Input: part model. Units: mm. Frame: model coordinates. Face numbers are marked on the shaded views. A direction names the side the tool comes from. Coordinates: 2 decimals unless noted, no trailing zeros. Loops run counter-clockwise (first coordinate to the right, second up) from the corner with the lowest first, then second, coordinate; pieces in that order, holes last. Notation, with made-up numbers: (48, -26) -> (94, -26) arc R20 cw to (94, -20) -> close; hole circle Ø3 at (16, -14.75). An arc over 180 degrees is marked (long way). Answer as a JSON object with one key per item and string values.
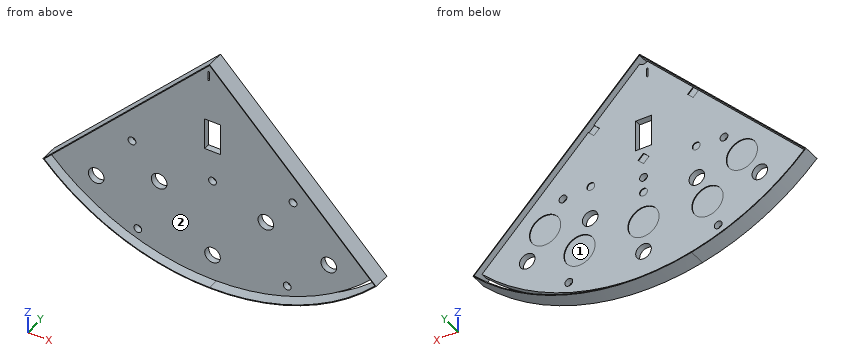
Autodesk Inventor part; units mm, degrees
ref_plane "YZ Plane" through (0, 0, 0) normal (1, 0, 0) x (0, 1, 0)
ref_plane "XZ Plane" through (0, 0, 0) normal (0, 1, 0) x (-1, 0, 0)
ref_plane "XY Plane" through (0, 0, 0) normal (0, 0, 1) x (1, 0, 0)
sketch "草圖1" plane through (0, 0, 0) normal (0, 1, 0) x (-1, 0, 0)
  line L0 (0, 0) -> (-1060.6602, -1060.6602)
  arc A0 (-1060.6602, -1060.6602) -> (0, -1500) centre (0, 0) ccw
  line L1 (0, -1500) -> (0, 0)
  line L2 (0, 0) -> (1060.6602, -1060.6602)
  arc A1 (0, -1500) -> (1060.6602, -1060.6602) centre (0, 0) ccw
  line L3 (1067.7254, -1060.6543) -> (0, 7.0711)
  line L4 (0, 7.0711) -> (-1067.7254, -1060.6543)
  arc A2 (-1067.7254, -1060.6543) -> (333.9619, -1467.4789) centre (0, 0) ccw
  arc A3 (333.9619, -1467.4789) -> (1067.7254, -1060.6543) centre (0, 0) ccw
  arc A4 (-1035.9114, -1035.9114) -> (332.6512, -1426.7334) centre (0, 0) ccw
  arc A5 (332.6512, -1426.7334) -> (1035.9114, -1035.9114) centre (0, 0) ccw
  line L5 (1549.2947, 0) -> (-1565.2813, 0)
  arc A6 (-24.7487, -24.7487) -> (24.7487, -24.7487) centre (0, 0) ccw
  line L6 (25, -130) -> (25, -70) construction
  line L7 (30, -125) -> (30, -75)
  line L8 (20, -75) -> (20, -125)
  arc A7 (20, -125) -> (30, -125) centre (25, -125) ccw
  arc A8 (30, -75) -> (20, -75) centre (25, -75) ccw
  line L9 (50, -400) -> (-50, -400)
  line L10 (-50, -400) -> (-50, -600)
  line L11 (-50, -600) -> (50, -600)
  line L12 (50, -600) -> (50, -400)
  line L13 (50, -400) -> (-50, -600) construction
  line L14 (-50, -400) -> (50, -600) construction
  point P0 (-7.0711, 0)
  point P1 (7.0711, 0)
  point P2 (24.7487, -682.358)
  point P3 (-24.7487, -682.358)
  point P4 (353.5534, -353.5534)
  point P5 (353.5534, -353.5534)
  point P6 (-353.5534, -353.5534)
  point P7 (-353.5534, -353.5534)
  point P8 (-7.0711, 0)
  point P9 (7.0711, 0)
  point P10 (25, -100)
  point P11 (0, -500)
  dimension "d0" = 1500
  dimension "d2" = 5
  dimension "d3" = 35
  dimension "d7" = 45
  dimension "d8" = 35
  dimension "d26" = 5
  dimension "d27" = 50
  dimension "d28" = 100
  dimension "d29" = 50
  dimension "d32" = 100
  dimension "d33" = 200
  dimension "d39" = 300
extrude "擠出1" add sketch "草圖1" along normal blind 40 and the other way blind 70 contours L5 L4 L3 | L5 L3 A3 A2 L4
extrude "擠出2" add sketch "草圖1" against normal blind 40 contours A6 L1 L9 L10 L11 A4 L0 | A6 L2 A5 A4 L1 L11 L12 L9
sketch "草圖2" plane through (0, 0, 0) normal (0, 1, 0) x (-1, 0, 0)
  line L0 (353.5534, -353.5534) -> (0, -707.1068) construction
  line L1 (0, -707.1068) -> (-353.5534, -353.5534) construction
  line L2 (-353.5534, -353.5534) -> (0, 0) construction
  line L3 (0, 0) -> (353.5534, -353.5534) construction
  line L4 (0, -707.1068) -> (35.3553, -671.7514)
  line L5 (35.3553, -671.7514) -> (0, -636.3961)
  line L6 (0, -636.3961) -> (-35.3553, -671.7514)
  line L7 (-35.3553, -671.7514) -> (0, -707.1068)
  line L8 (318.1981, -388.9087) -> (353.5534, -353.5534)
  line L9 (353.5534, -353.5534) -> (318.1981, -318.1981)
  line L10 (318.1981, -318.1981) -> (282.8427, -353.5534)
  line L11 (282.8427, -353.5534) -> (318.1981, -388.9087)
  line L12 (-318.1981, -388.9087) -> (-282.8427, -353.5534)
  line L13 (-282.8427, -353.5534) -> (-318.1981, -318.1981)
  line L14 (-318.1981, -318.1981) -> (-353.5534, -353.5534)
  line L15 (-353.5534, -353.5534) -> (-318.1981, -388.9087)
  line L16 (-1060.6602, -1060.6602) -> (0, 0)
  line L17 (0, 0) -> (1060.6602, -1060.6602)
  arc A0 (-24.7487, -24.7487) -> (24.7487, -24.7487) centre (0, 0) ccw
  dimension "d15" = 500
  dimension "d19" = 50
  dimension "d20" = 50
  dimension "d21" = 50
extrude "擠出3" cut sketch "草圖2" against normal blind 5 contours L7 L6 L5 L4 | L11 L10 L9 L8 | L13 L12 L15 L14
sketch "草圖6" plane through (0, 0, 0) normal (0, 1, 0) x (1, 0, 0)
  line L0 (0, 0) -> (1060.6602, 1060.6602)
  line L1 (-1067.7254, 1060.6543) -> (0, -7.0711)
  arc A0 (919.2388, 919.2388) -> (-922.7676, 915.6965) centre (0, 0) ccw construction
  line L2 (0, 0) -> (-1060.6602, 1060.6602)
  arc A1 (777.8175, 777.8175) -> (-777.8175, 777.8175) centre (0, 0) ccw construction
  arc A2 (636.3961, 636.3961) -> (-634.8813, 637.9073) centre (0, 0) ccw construction
  circle A3 centre (0, 1300) radius 50
  arc A4 (1035.9114, 1035.9114) -> (-1035.9114, 1035.9114) centre (0, 0) ccw
  line L3 (0, 1465) -> (0, 0) construction
  circle A5 centre (0, 1100) radius 100
  circle A6 centre (0, 900) radius 25
  circle A7 centre (-745.6494, 1064.8977) radius 50
  circle A8 centre (-630.9341, 901.0672) radius 100
  circle A9 centre (-516.2188, 737.2368) radius 25
  circle A10 centre (745.6494, 1064.8977) radius 50
  circle A11 centre (630.9341, 901.0672) radius 100
  circle A12 centre (516.2188, 737.2368) radius 25
  arc A13 (989.9495, 989.9495) -> (-993.7497, 986.1347) centre (0, 0) ccw construction
  arc A14 (848.5281, 848.5281) -> (-848.5281, 848.5281) centre (0, 0) ccw construction
  arc A15 (707.1068, 707.1068) -> (-705.4236, 708.7859) centre (0, 0) ccw construction
  line L4 (0, 0) -> (501.0595, 1376.6497) construction
  circle A16 centre (342.0201, 939.6926) radius 50
  circle A17 centre (478.8282, 1315.5697) radius 25
  circle A18 centre (410.4242, 1127.6311) radius 100
  circle A19 centre (-342.0201, 939.6926) radius 50
  circle A20 centre (-478.8282, 1315.5697) radius 25
  circle A21 centre (-410.4242, 1127.6311) radius 100
  arc A22 (565.6854, 565.6854) -> (-565.6854, 565.6854) centre (0, 0) ccw construction
  circle A23 centre (0, 800) radius 25
  circle A24 centre (-338.0946, 725.0462) radius 25
  circle A25 centre (338.0946, 725.0462) radius 25
  point P0 (0, 1100)
  dimension "d44" = 1300
  dimension "d45" = 1100
  dimension "d46" = 900
  dimension "d47" = 100
  dimension "d48" = 200
  dimension "d49" = 50
  dimension "d52" = 35
  dimension "d54" = 100
  dimension "d55" = 100
  dimension "d56" = 100
  dimension "d57" = 25
  dimension "d58" = 100
  dimension "d59" = 50
  dimension "d60" = 200
  dimension "d63" = 100
  dimension "d66" = 50
  dimension "d69" = 25
extrude "擠出6" cut sketch "草圖6" against normal blind 5 contours A5 | A6 | A8 | A11 | A18 | A21 | A24 | A25
extrude "擠出7" cut sketch "草圖6" against normal through all contours A3 | A7 | A9 | A10 | A12 | A16 | A17 | A19 | A20 | A23
properties part number "球場2"
1. Pin query (flat end, axial travel): P1, Ø1, axis at x = -202, z = -468.5, coming from the -Y side; P2, Ø5, axis at y = -44.5, z = -1148, coming from the +X side; P3, Ø8, axis at x = 230, y = 3, coming from the +Z side. Return the tip coordinate at first contact, or that it passes through.
Reply:
{"P1": "stops at y = -40", "P2": "stops at x = 976.14", "P3": "stops at z = -218.93"}
2. Section query A-A (z = -487.5). Return loops of the section in (x, y).
Reply:
{"outline": "(-494.57, -70) -> (-487.5, -70) -> (-487.5, -40) -> (-50, -40) -> (-50, 0) -> (-487.5, 0) -> (-487.5, 40) -> (-494.57, 40) -> close; (50, -40) -> (487.5, -40) -> (487.5, -70) -> (494.57, -70) -> (494.57, 40) -> (487.5, 40) -> (487.5, 0) -> (50, 0) -> close"}
3. Access query for the marked faces 1 and 2. Directions: +Z, -Z, +X, -X, +Y, -Y. A direction counts if a zero-diameter tool reaches every point of the face in a straight line with its end or side. Return the directions, or none.
Reply:
{"face 1": "+Y", "face 2": "-Y"}
4. Section query C-C (z = -1149). Return loops of the section in (x, y).
Reply:
{"outline": "(-972.02, -70) -> (-964.26, -70) -> (-964.26, 40) -> (-972.02, 40) -> close; (-908.86, -40) -> (908.86, -40) -> (908.86, 0) -> (508.11, 0) -> (508.11, -5) -> (312.73, -5) -> (312.73, 0) -> (87.17, 0) -> (87.17, -5) -> (-87.17, -5) -> (-87.17, 0) -> (-312.73, 0) -> (-312.73, -5) -> (-508.11, -5) -> (-508.11, 0) -> (-908.86, 0) -> close; (964.26, -70) -> (972.02, -70) -> (972.02, 40) -> (964.26, 40) -> close"}
5. Line query: line 1 along Z through (x, y) = (-754.5, -4); line 2 along X through (y, z) = (-32, -1020.5); line 3 along Z through (x, y) = (-705, -2). Output: solid intervals per line, ascending.
Reply:
{"line 1": "z = -1302.21 to -1296.43, -1255.77 to -1114.11, -1015.69 to -747.43", "line 2": "x = -1027.57 to -768.65, -722.65 to 722.65, 768.65 to 1027.57", "line 3": "z = -1329.66 to -1324, -1284.21 to -1094.01, -1035.78 to -968.26, -833.88 to -697.93"}
6. Section query B-B (x = -202.5). Return loops of the section in (y, z).
Reply:
{"outline": "(-70, -1491.31) -> (40, -1491.31) -> (40, -1486.27) -> (-70, -1486.27) -> close; (-70, -202.5) -> (-40, -202.5) -> (-40, -1450.94) -> (0, -1450.94) -> (0, -202.5) -> (40, -202.5) -> (40, -195.43) -> (-70, -195.43) -> close"}
